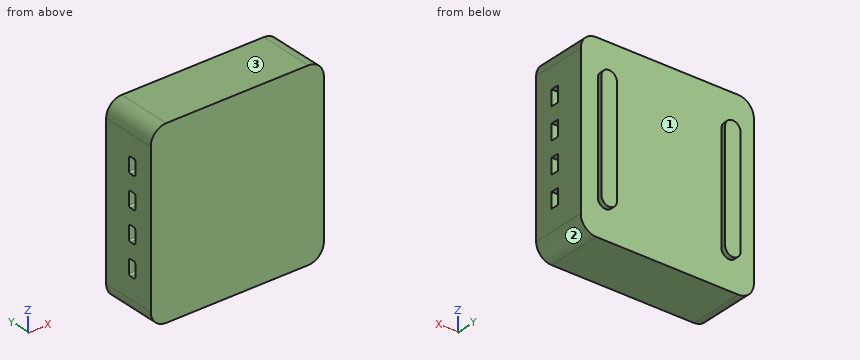
```python
from build123d import *

# Parameters (mm, degrees)
SKETCH_1_W          = 112
SKETCH_1_H          = 117
EXTRUDE_1_DEPTH     = 36
FILLET_1_R          = 10
EXTRUDE_2_DEPTH     = 3
SKETCH_4_W          = 10
SKETCH_4_H          = 5
CUT_EXTRUDE_1_DEPTH = 10
FILLET_2_R          = 1
SKETCH_5_W          = 10
SKETCH_5_H          = 5
CUT_EXTRUDE_2_DEPTH = 10


with BuildPart() as part:
    # 草图1 → 凸台-拉伸1 (new body)
    with BuildSketch(Plane(origin=(0, 0, 0), x_dir=(1, 0, 0), z_dir=(0, 1, 0))):
        Rectangle(SKETCH_1_W, SKETCH_1_H)
    extrude(amount=EXTRUDE_1_DEPTH)

    # 圆角1
    fillet_1_edges = [part.edges().sort_by_distance(p)[0] for p in [
        (56, 18, 58.5),
        (-56, 18, 58.5),
        (-56, 18, -58.5),
        (56, 18, -58.5),
    ]]
    fillet(fillet_1_edges, radius=FILLET_1_R)

    # 草图3 → 凸台-拉伸2 (add)
    with BuildSketch(Plane(origin=(0, 36, 0), x_dir=(1, 0, 0), z_dir=(0, 1, 0))):
        with BuildLine():
            Line((-35, 35), (-35, -35))
            ThreePointArc((-35, -35), (-40, -40), (-45, -35))
            Line((-45, -35), (-45, 35))
            ThreePointArc((-45, 35), (-40, 40), (-35, 35))
        make_face()
        with BuildLine():
            Line((35, 35), (35, -35))
            ThreePointArc((35, -35), (40, -40), (45, -35))
            Line((45, -35), (45, 35))
            ThreePointArc((45, 35), (40, 40), (35, 35))
        make_face()
    extrude(amount=EXTRUDE_2_DEPTH)

    # 草图4 → 切除-拉伸1 (cut)
    with BuildSketch(Plane.ZY.offset(56)):
        with Locations((-10, 15)):
            Rectangle(SKETCH_4_W, SKETCH_4_H)
        with Locations((-30, 15)):
            Rectangle(SKETCH_4_W, SKETCH_4_H)
        with Locations((10, 15)):
            Rectangle(SKETCH_4_W, SKETCH_4_H)
        with Locations((30, 15)):
            Rectangle(SKETCH_4_W, SKETCH_4_H)
    extrude(amount=-CUT_EXTRUDE_1_DEPTH, mode=Mode.SUBTRACT)

    # 圆角2
    fillet_2_edges = [part.edges().sort_by_distance(p)[0] for p in [
        (-51, 12.5, -35),
        (-51, 17.5, -35),
        (-51, 17.5, -25),
        (-51, 12.5, -25),
        (-51, 17.5, -15),
        (-51, 17.5, -5),
        (-51, 12.5, -5),
        (-51, 12.5, -15),
        (-51, 17.5, 5),
        (-51, 17.5, 15),
        (-51, 12.5, 15),
        (-51, 12.5, 5),
        (-51, 17.5, 25),
        (-51, 17.5, 35),
        (-51, 12.5, 35),
        (-51, 12.5, 25),
    ]]
    fillet(fillet_2_edges, radius=FILLET_2_R)

    # 草图5 → 切除-拉伸2 (cut)
    with BuildSketch(Plane(origin=(56, 0, 0), x_dir=(0, 0, -1), z_dir=(1, 0, 0))):
        with Locations((-10, 15)):
            Rectangle(SKETCH_5_W, SKETCH_5_H)
        with Locations((-30, 15)):
            Rectangle(SKETCH_5_W, SKETCH_5_H)
        with Locations((10, 15)):
            Rectangle(SKETCH_5_W, SKETCH_5_H)
        with Locations((30, 15)):
            Rectangle(SKETCH_5_W, SKETCH_5_H)
    extrude(amount=-CUT_EXTRUDE_2_DEPTH, mode=Mode.SUBTRACT)


solid = part.part
```
Read the model definition and answer for the solid it produces. Units are mm, in the model's axes. Face numbers are marked on the shaded views. Give positions to 0.01 mm unless a question says otherwise; leave off trailing zeros. Order: outer loops, then holes, each group sorted by start corner. A loop starts at its lowest first (then second) coordinate and runs counter-clockwise, first axis right, second up. Notation, with made-up numbers: (7, -37) -> (33, -37) arc R15 ccw to (33, -12) -> close; hole circle Ø5 at (8.5, 81). An arc over 180 degrees is marked (long way). One line per item, written item: value. Start each with the question number.
(1) The part is cut by section D-D (x = 16). Determine the outline of the cut face in (y, z).
(2) Straight lines are drawn through the part: L1, parallel to X at y = 36.5, z = -23.5; L2, parallel to X at y = 13, z = -26; L3, parallel to Y at x = 45.5, z = -36.5. For each, find the intervals that lie inside material, in ascending order.
(3) For a pull along X with two mould halves and no side action, classify the marked faces 1, 2 and 3 as released by +X, released by -X, zero draft, split by the parting line, or undercut.
(4) The part is cut by section A-A (z = 28). Determine the outline of the cut face in (x, y), and give its area (3 significant figures).
(5) Flat-ended cylindrical pins translate along their axes: P1, Ø3, axis at x = 52.5, z = -10, coming from the +Y side; P2, Ø1.5, axis at x = -51, y = 14.5, coming from the -Z side; P3, Ø2.5, axis at x = -52, y = 15.5, coming from the +Z side. Find the tip coordinate at first contact, or state that the pin passes through.
(6) The part is cut by section C-C (z = -22). Determine the outline of the cut face in (x, y).
(7) The part is cut by section B-B (x = -40). Determine the outline of the cut face in (y, z).
Taken from the geometry:
1. outline: (0, -58.5) -> (36, -58.5) -> (36, 58.5) -> (0, 58.5) -> close
2. L1: -45 to -35, 35 to 45
2. L2: -46 to 46
2. L3: 0 to 36
3. face 1: undercut
3. face 2: released by +X
3. face 3: zero draft
4. outline: (-56, 0) -> (56, 0) -> (56, 12.5) -> (46, 12.5) -> (46, 17.5) -> (56, 17.5) -> (56, 36) -> (45, 36) -> (45, 39) -> (35, 39) -> (35, 36) -> (-35, 36) -> (-35, 39) -> (-45, 39) -> (-45, 36) -> (-56, 36) -> (-56, 17.5) -> (-46, 17.5) -> (-46, 12.5) -> (-56, 12.5) -> close
4. area: 3,990 mm^2
5. P1: y = 36
5. P2: z = -57.55
5. P3: z = 57.3
6. outline: (-56, 0) -> (56, 0) -> (56, 36) -> (45, 36) -> (45, 39) -> (35, 39) -> (35, 36) -> (-35, 36) -> (-35, 39) -> (-45, 39) -> (-45, 36) -> (-56, 36) -> close
7. outline: (0, -58.5) -> (36, -58.5) -> (36, -40) -> (39, -40) -> (39, 40) -> (36, 40) -> (36, 58.5) -> (0, 58.5) -> close
